Autodesk Inventor part; units mm, degrees
ref_plane "YZ Plane" through (0, 0, 0) normal (1, 0, 0) x (0, 1, 0)
ref_plane "XZ Plane" through (0, 0, 0) normal (0, 1, 0) x (-1, 0, 0)
ref_plane "XY Plane" through (0, 0, 0) normal (0, 0, 1) x (1, 0, 0)
sketch "Boceto1" plane through (0, 0, 0) normal (0, 1, 0) x (-1, 0, 0)
  line L0 (-85, -175) -> (85, -175)
  line L1 (85, -175) -> (85, 175)
  line L2 (85, 175) -> (-85, 175)
  line L3 (-85, 175) -> (-85, -175)
  line L4 (70, 160) -> (70, -160)
  line L5 (85, -160) -> (-85, -160)
  line L6 (-70, -160) -> (-70, 160)
  line L7 (-85, 160) -> (85, 160)
  line L8 (0, -160) -> (0, -60) construction
  line L9 (0, 175) -> (0, 29.19) construction
  circle A0 centre (0, 29.19) radius 5 construction
  line L10 (0, 29.19) -> (0, 0.69) construction
  line L11 (0, 29.19) -> (0, 57.69) construction
  line L12 (17.8997, 57.69) -> (-17.8997, 57.69) construction
  line L13 (-17.8997, 57.69) -> (-17.8997, 0.69) construction
  line L14 (-17.8997, 0.69) -> (17.8997, 0.69) construction
  line L15 (17.8997, 0.69) -> (17.8997, 57.69) construction
  point P0 (0, 0)
  dimension "d0" = 170
  dimension "d1" = 350
  dimension "d2" = 15
  dimension "d7" = 100
  dimension "d8" = 145.81
  dimension "d9" = 10
  dimension "d12" = 28.5
  dimension "d13" = 28.5
extrude "Extrusión1" add sketch "Boceto1" along normal blind 100 contours L3 L5 L1 L0
extrude "Extrusión2" add sketch "Boceto1" along normal blind 100 contours L5 L4 L7 L1
extrude "Extrusión3" add sketch "Boceto1" against normal blind 15
sketch "Boceto2" plane through (-70, 100, -160) normal (0, 0, 1) x (1, 0, 0)
  line L0 (155, -100) -> (155, 0) construction
  line L1 (0, 0) -> (77.5, 0)
  line L2 (0, 0) -> (155, 0)
  line L3 (77.5, -100) -> (70, -100) construction
  line L4 (0, -100) -> (155, -100) construction
  line L5 (70, -100) -> (70, -74.5) construction
  circle A0 centre (70, -74.5) radius 2.5
  circle A1 centre (70, -74.5) radius 7.5
  dimension "d94" = 7.5
  dimension "d95" = 25.5
  dimension "d96" = 5
  dimension "d97" = 5
extrude "Extrusión4" cut sketch "Boceto2" against normal through all contours A0
extrude "Extrusión5" add sketch "Boceto1" along normal blind 100 contours L3 L2 L1 L7
extrude "Extrusión6" add sketch "Boceto1" along normal blind 100 contours L3 L7 L6 L5
sketch "Boceto3" plane through (0, 0, 0) normal (0, 1, 0) x (1, 0, 0)
  line L0 (-70, -160) -> (-70, 160) construction
  line L1 (-70, -160) -> (7.5, -160) construction
  line L2 (-70, -160) -> (85, -160) construction
  line L3 (-70, -160) -> (7.5, -160) construction
  line L4 (7.5, -29.19) -> (-9, -29.19) construction
  line L5 (15, -57.69) -> (5.97, -57.69)
  line L6 (5.97, -57.69) -> (5.97, -48.59)
  line L7 (5.97, -48.59) -> (15, -48.59)
  line L8 (15, -48.59) -> (15, -57.69)
  line L9 (15, -0.69) -> (7.47, -0.69)
  line L10 (7.47, -0.69) -> (7.47, -13.65)
  line L11 (7.47, -13.65) -> (15, -13.65)
  line L12 (15, -13.65) -> (15, -0.69)
  line L13 (85, 175) -> (85, -175)
  line L14 (85, -29.19) -> (0, -29.19) construction
  circle A0 centre (0, -29.19) radius 3.5
  line L15 (0, -29.19) -> (0, -22.225) construction
  line L16 (-15, -57.69) -> (-5.97, -57.69)
  line L17 (-5.97, -48.59) -> (-15, -48.59)
  line L18 (-15, -48.59) -> (-15, -57.69)
  line L19 (-15, -0.69) -> (-7.47, -0.69)
  line L20 (-7.47, -0.69) -> (-7.47, -13.65)
  line L21 (-7.47, -13.65) -> (-15, -13.65)
  line L22 (-15, -13.65) -> (-15, -0.69)
  line L23 (-5.97, -57.69) -> (-5.97, -48.59)
  line L24 (-85, -175) -> (85, -175)
  point P0 (-85, -160)
  point P1 (15, -7.17)
  point P2 (-15, -7.17)
  dimension "d46" = 9.03
  dimension "d47" = 9.1
  dimension "d48" = 12.96
  dimension "d54" = 85
  dimension "d55" = 7
  dimension "d62" = 30
  dimension "d63" = 30
  dimension "d68" = 70
  dimension "d69" = 117.31
  dimension "d70" = 90.97
  dimension "d71" = 161.35
  dimension "d72" = 70
  dimension "d73" = 7.53
  dimension "d74" = 92.47
extrude "Extrusión12" cut sketch "Boceto3" against normal blind 5 contours L5 L6 L7 L8 | L12 L11 L10 L9 | L18 L17 L23 L16 | L19 L20 L21 L22
extrude "Extrusión13" cut sketch "Boceto3" against normal through all contours A0
sketch "Boceto8" plane through (85, 100, -160) normal (1, 0, 0) x (0, 0, -1)
  line L0 (-320, -100) -> (0, -100)
  line L1 (0, -100) -> (-100, -100)
  line L2 (-100, -100) -> (-100, -14.2875)
  line L3 (-335, -100) -> (0, -100)
  line L4 (-192.69, -100) -> (-185.69, -100)
  line L5 (-189.19, -100) -> (-100, -100)
  line L6 (-335, -115) -> (15, -115)
  point P0 (-160, -100)
  dimension "d66" = 100
  dimension "d67" = 89.19
sketch "Boceto9" plane through (0, 0, 0) normal (0, 1, 0) x (1, 0, 0)
  line L0 (0, 160) -> (0, 60)
  line L1 (0, 60) -> (40, 60) construction
  line L2 (0, 60) -> (-40, 60) construction
  line L3 (0, 60) -> (-40, 60) construction
  line L4 (40, 60) -> (40, 52.5) construction
  line L5 (40, 60) -> (40, 67.5) construction
  line L6 (40, 67.5) -> (20, 67.5)
  line L7 (20, 67.5) -> (20, 52.5)
  line L8 (20, 52.5) -> (40, 52.5)
  line L9 (40, 52.5) -> (40, 67.5)
  line L10 (-40, 60) -> (-40, 67.5) construction
  line L11 (-40, 67.5) -> (-20, 67.5)
  line L12 (-20, 67.5) -> (-20, 52.5)
  line L13 (-20, 52.5) -> (-40, 52.5)
  line L14 (-40, 67.5) -> (-40, 52.5)
  line L15 (-20, 80) -> (-40, 80)
  line L16 (-40, 80) -> (-40, 40)
  line L17 (-40, 40) -> (-20, 40)
  line L18 (-20, 40) -> (-20, 80)
  line L19 (20, 80) -> (40, 80)
  line L20 (40, 80) -> (40, 40)
  line L21 (40, 40) -> (20, 40)
  line L22 (20, 40) -> (20, 80)
  point P0 (0, 0)
  point P1 (-30, 60)
  dimension "d80" = 100
  dimension "d83" = 40
  dimension "d86" = 7.5
  dimension "d87" = 7.5
  dimension "d88" = 20
  dimension "d89" = 15
  dimension "d98" = 20
  dimension "d99" = 40
extrude "Extrusión14" [suppressed]
sketch "Boceto10" plane through (0, 0, 0) normal (0, 1, 0) x (1, 0, 0)
  circle A0 centre (0, -29.19) radius 3.5
  line L0 (0, -29.19) -> (0, 170.81)
  line L1 (0, -29.19) -> (200, -29.19) construction
  point P0 (0, 0)
  dimension "d92" = 200
  dimension "d93" = 90
extrude "Extrusión15" [suppressed]
properties part number "DarkBox" material "Madera (cerezo)"
Geometry: final body of the model. Coordinates: model frame, mm. A direction names the side the tool comes from. Round coordinates to 2 decimals unless told otherwise and drop trailing zeros. Write each loop counter-clockwise with the first axis right and the second up, starting at its lowest first coordinate (ties: lowest second). Pieces come first, ordered by that corner, then holes.
Item 1: Section query D-D (z = -111). Return loops of the section in (x, y), plus the area to 3 significant figures.
Item 2: Section query A-A (y = 18). Return loops of the section in (x, z).
Item 3: Section query B-B (z = 29.19). Return loops of the section in (x, y), plus the area to 4 significant figures.
Item 4: Pin query (flat end, axial travel): P1, Ø1.5, axis at x = 14.5, z = -49, coming from the +Y side; P2, Ø2.5, axis at x = 10.5, z = 4, coming from the +Y side; P3, Ø6.5, axis at x = 0, y = 25.5, coming from the -Z side. Return the tip coordinate at first contact, or that it passes through.
Item 5: Material intervals for L1, parallel to X at y = 52.5, z = -25; L2, parallel to Z at x = 0, y = -8; L3, parallel to Z at x = 39, y = 62, sorted ascending.
Item 6: Mould query, pull axis X, two halves, no side actions, for faces 3 (the face through (76, 100, 14)), 4 (the face through (1, 0, 2)), 5 (the face through (-1, 49, -160)), 6 (the face through (85, 42, 2)). Classes: +X half, -X half, draft (parallel to the pull), parting line (faces both ways), or undercut.
Item 7: Section query C-C (x = -40). Return loops of the section in (y, z).
Item 8: Set-up query: faces 1 (the face through (11, -5, 7)), 2 (the face through (-1, 42, 175)). Return all of +Z, -Z, +X, -X, +Y, -Y with unobstructed straight access to the full face (end or side cutting, diameter ignored); none if empty.
Completed:
1. outline: (-85, -15) - (85, -15) - (85, 100) - (70, 100) - (70, 0) - (-70, 0) - (-70, 100) - (-85, 100) - close
1. area: 5,550 mm2
2. outline: (-85, -175) - (85, -175) - (85, 175) - (-85, 175) - close; hole (-70, -160) - (70, -160) - (70, 160) - (-70, 160) - close
3. outline: (-85, -15) - (-3.5, -15) - (-3.5, 0) - (-70, 0) - (-70, 100) - (-85, 100) - close; (3.5, -15) - (85, -15) - (85, 100) - (70, 100) - (70, 0) - (3.5, 0) - close
3. area: 5,445 mm2
4. P1: stops at y = 0
4. P2: stops at y = -5
4. P3: stops at z = -175
5. L1: x = -85 to -70, 70 to 85
5. L2: z = -175 to 25.69, 32.69 to 175
5. L3: z = -175 to -160, 160 to 175
6. face 3: draft
6. face 4: undercut
6. face 5: undercut
6. face 6: +X half
7. outline: (-15, -175) - (100, -175) - (100, -160) - (0, -160) - (0, 160) - (100, 160) - (100, 175) - (-15, 175) - close
8. face 1: +Y
8. face 2: +Z, +X, -X, +Y, -Y
